from build123d import *

# Parameters (mm, degrees)
CUT_EXTRUDE1_DEPTH      = 17.064109466
CUT_EXTRUDE1_DEPTH_BACK = 17.064109466
SKETCH2_W               = 2.159
SKETCH2_H               = 5.314367205
CUT_EXTRUDE2_DEPTH      = 17.064109466
CUT_EXTRUDE2_DEPTH_BACK = 17.064109466
SKETCH3_R               = 0.4445
BOSS_EXTRUDE8_START     = -0.508
SKETCH4_R               = 2.5908
SKETCH4_R_2             = 1.9558
BOSS_EXTRUDE8_DEPTH     = 0.508
FILLET1_R               = 2.54


with BuildPart() as part:
    # Sketch1 one side → Revolve1 (revolve)
    with BuildSketch(Plane.XY):
        with BuildLine():
            Line((1.9558, -13.8684), (1.9558, 0))
            ThreePointArc((1.9558, 0), (1.382959443, 1.382959443), (0, 1.9558))
            Line((0, 1.9558), (0, -15.8242))
            ThreePointArc((0, -15.8242), (1.382959443, -15.251359443), (1.9558, -13.8684))
        make_face()
    revolve(axis=Axis((0, 0, 0), (0, -1, 0)))

    # Sketch2 → Cut-Extrude1 (cut, two sides: drawn at the far end of the back side and taken through both)
    with BuildSketch(Plane(origin=(0, 0, 0), x_dir=(0, 0, -1), z_dir=(1, 0, 0)).offset(-CUT_EXTRUDE1_DEPTH_BACK)):
        with Locations((0, -0.517816398)):
            Rectangle(SKETCH2_W, SKETCH2_H)
    extrude(amount=CUT_EXTRUDE1_DEPTH + CUT_EXTRUDE1_DEPTH_BACK, mode=Mode.SUBTRACT)

    # Sketch3 → Cut-Extrude2 (cut, two sides: drawn at the far end of the back side and taken through both)
    with BuildSketch(Plane.XY.offset(-CUT_EXTRUDE2_DEPTH_BACK)):
        Circle(SKETCH3_R)
    extrude(amount=CUT_EXTRUDE2_DEPTH + CUT_EXTRUDE2_DEPTH_BACK, mode=Mode.SUBTRACT)

    # Sketch4 → Boss-Extrude8 (add)
    with BuildSketch(Plane(origin=(0, -13.8684, 0), x_dir=(-1, 0, 0), z_dir=(0, -1, 0)).offset(BOSS_EXTRUDE8_START)):
        with Locations(Location((0, 0, 0), (0, 0, 90))):
            Circle(SKETCH4_R)
        with Locations(Location((0, 0, 0), (0, 0, 213.500760385))):
            Circle(SKETCH4_R_2, mode=Mode.SUBTRACT)
    extrude(amount=BOSS_EXTRUDE8_DEPTH)

    # Fillet1
    # the kernel refuses this fillet: 2.54 mm, written as the material it adds along each edge
    with BuildSketch(Plane(origin=(0, -13.8684, 0), x_dir=(1, 0, 0), z_dir=(0, 0, -1))) as fillet1_piece_1:
        with BuildLine():
            CenterArc((3.951069608, 2.145056315), FILLET1_R, 208.497766198, 29.121746718)
            Line((2.5908, 0), (2.563594608, -0.042901126))
            ThreePointArc((2.563594608, -0.042901126), (2.2733, -0.0508), (1.9558, -0.0508))
            Line((1.9558, -0.0508), (1.905, 0))
            ThreePointArc((1.905, 0), (1.846394024, 0.46888603), (1.674182037, 0.908922167))
            Line((1.674182037, 0.908922167), (1.718826892, 0.933160092))
        make_face()
    revolve(axis=Axis((0, -13.8684, 0), (0, -1, 0)))


solid = part.part
The model under review builds one solid part; all positions refer to its coordinate system, in mm. A direction names the side the tool comes from. Coordinates: 2 decimals unless noted, no trailing zeros. Write each loop counter-clockwise with the first axis right and the second up, starting at its lowest first coordinate (ties: lowest second). Pieces come first, ordered by that corner, then holes. Notation, with made-up numbers: (51, 21) - (110, 21) arc R15 ccw to (110, 30) - close; hole circle Ø3 at (85, 2). An arc over 180 degrees is marked (long way). Answer as a JSON object with one key per item and string values. Group by question number.
1. To check wall thickness, follow probe 1 along Y at (x, z) = (0, -1.25); probe 2 along Z at (x, y) = (-0.1, -5.75); probe 3 along Y at (x, z) = (0, -1.65). State the ranges of each line that lie inside material, in increasing order.
2. Add section B-B (y = -0.25). Give the boundary of the cut face in (x, z), plus the area to 3 significant figures.
3. Mouldability with a two-part tool opening along Y and no side actions: class faces 1 (the face through (-0.096, -0.434, 1.513)), 2 (the face through (0, -3.175, 0)), 3 (the face through (-0.096, -0.434, -1.525)), 4 (the face through (0, -1, 1.08)) as pulls with the +Y half, pulls with the -Y half, needs draft (parallel to the pull), parting line crosses it, or undercut.
4. Clearance check with flat-ended pins moving along their axes: pin 1 Ø3 at (x, y) = (-1.5, -12) entering from -Z; pin 2 Ø1 at (x, y) = (-0.5, -0.5) entering from +Z; pin 3 Ø1 at (x, z) = (1.5, -1) entering from +Y; pin 4 Ø1.5 at (x, z) = (-0.5, 0.5) entering from -Y. State where each tip first meets the part, or that it passes through.
5. Add section D-D (y = -2.75). Give the boundary of the cut face in (x, z).
6. Add section A-A (x = 0). Give the boundary of the cut face in (y, z) (1 decimal).
7. Add section C-C (z = 0). Give the boundary of the cut face in (x, y) (3 decimals).
8. Machinability: for faces 5 (the face through (0, -1, -1.08)), 6 (the face through (0.78, -13.61, -2.47)), 7 (the face through (-1.954, -6.587, 0.086)), which of the approach directions +Z, -Z, +X, -X, +Y, -Y give a long, thin tool a straight path to every point of the face, cutting with its end or side? Answer none if there is none.
Findings:
{
 "1": {"probe 1": "-15.37 to -0.44, 0.44 to 1.5", "probe 2": "-1.95 to 1.95", "probe 3": "-14.92 to -0.44, 0.44 to 1.05"},
 "2": {"outline": "(-1.63, -1.08) arc R1.96 ccw to (-0.37, -1.92) - (-0.37, -1.08) - close; (-1.63, 1.08) - (-0.37, 1.08) - (-0.37, 1.92) arc R1.96 ccw to start; (0.37, -1.92) arc R1.96 ccw to (1.63, -1.08) - (0.37, -1.08) - close; (0.37, 1.08) - (1.63, 1.08) arc R1.96 ccw to (0.37, 1.92) - close", "area": "2.75 mm²"},
 "3": {"face 1": "undercut", "face 2": "pulls with the +Y half", "face 3": "undercut", "face 4": "needs draft"},
 "4": {"pin 1": "z = -2.44", "pin 2": "z = 1.96", "pin 3": "y = 1.28", "pin 4": "y = -15.82"},
 "5": {"outline": "(-1.63, -1.08) arc R1.96 ccw to (1.63, -1.08) - close; (-1.63, 1.08) - (1.63, 1.08) arc R1.96 ccw to start"},
 "6": {"outline": "(-14.8, -1.7) arc R2.5 cw to (-13.9, -2.6) - (-13.4, -2.6) - (-13.4, -2) - (-0.4, -2) - (-0.4, -1.1) - (-3.2, -1.1) - (-3.2, 1.1) - (-0.4, 1.1) - (-0.4, 2) - (-13.4, 2) - (-13.4, 2.6) - (-13.9, 2.6) arc R2.5 cw to (-14.8, 1.7) arc R2 ccw to start; (0.4, -1.9) arc R2 ccw to (1.6, -1.1) - (0.4, -1.1) - close; (0.4, 1.1) - (1.6, 1.1) arc R2 ccw to (0.4, 1.9) - close"},
 "7": {"outline": "(-2.591, -13.868) arc R2.54 cw to (-1.719, -14.802) arc R1.956 ccw to (1.719, -14.802) arc R2.54 cw to (2.591, -13.868) - (2.591, -13.36) - (1.956, -13.36) - (1.956, -3.175) - (-1.956, -3.175) - (-1.956, -13.36) - (-2.591, -13.36) - close"},
 "8": {"face 5": "+X, -X, +Y", "face 6": "+Y, -Y", "face 7": "+Y"}
}
